```python
from build123d import *


with BuildPart() as f1:
    # F0 (on Front) → F1 (revolve)
    with BuildSketch(Plane.XZ):
        with BuildLine():
            Line((0, 50), (0, 0))
            Line((0, 0), (172.990381, 0))
            Line((172.990381, 0), (160, 7.5))
            Line((160, 7.5), (160, 2.5))
            Line((160, 2.5), (155, 2.5))
            Line((155, 2.5), (22.421579, 75.891626))
            ThreePointArc((22.421579, 75.891626), (17.461092, 75.824589), (15, 71.51716))
            Line((15, 71.51716), (15, 50))
            Line((15, 50), (0, 50))
        make_face()
    revolve(axis=Axis((-26.037737, 0, 0), (-1, 0, 0)))


solid = f1.part
```
Can you work these out from the model? Positions are in its coordinate system, mm. A direction names the side the tool comes from. Coordinates: 2 decimals unless noted, no trailing zeros. Loops run counter-clockwise (first coordinate to the right, second up) from the corner with the lowest first, then second, coordinate; pieces in that order, holes last. Notation, with made-up numbers: (14.5, 69.5) - (20.5, 69.5) arc R11 cw to (20.5, 90.5) - close; hole circle Ø4 at (68, 1.5). An arc over 180 degrees is marked (long way). Answer as CSV lines item,"result". Start each with the question number.
1) Thinking about a two-plate mould opening in X: for faces 1 (the cylindrical face through (7.4, 15.02, 47.69)), 2 (the flat face through (15, 49, 15)), 3 (the flat face through (160, 2, -2)), which applies, pulls with the +X half, pulls with the -X half, needs draft (parallel to the pull), parting line crosses it, or undercut?
2) Which directions (+Z, -Z, +X, -X, +Y, -Y) give clear straight access to the entire face, cutting with the end or side of a thin tool? Please do faces 4 (the flat face through (0, 1, -1)), 5 (the cylindrical face through (157.46, -2.44, -0.54)).
3) Suppose I cut it at B-B (x = 149.5). Please give me the cut outline in (y, z).
4) Suppose I cut it at A-A (x = 56). Please give me the cut outline in (y, z), plus the area to 3 significant figures.
5) For pin 1 (7.5 mm diameter, centred on y = 1, z = -1.5, fed in from -X); pin 2 (1.5 mm diameter, centred on y = -35.5, z = 22, fed in from +X); pin 3 (12 mm diameter, centred on x = 61.5, y = 45, fed in from +Z); pin 4 (1 mm diameter, centred on x = 19.5, z = -45.5, fed in from -Y), each with a flat end and sliding along its axis, tell me the tip position at first contact or that it passes through.
6) I need wall thicknesses on line 1 (Y direction, x = 128, z = -0.5); line 2 (Y direction, x = 38, z = 19); line 3 (Z direction, x = 131, y = -0.5). Which ranges of each line are inside material? Lowest first, please. Write a range as from..to.
Check result:
1,face 1,"needs draft"
1,face 2,"pulls with the -X half"
1,face 3,"undercut"
2,face 4,"+Z, -Z, -X, +Y, -Y"
2,face 5,"none"
3,outline,"circle Ø11.09 at (0, 0)"
4,outline,"circle Ø114.61 at (0, 0)"
4,area,"10,300 mm²"
5,pin 1,"stops at x = 0"
5,pin 2,"stops at x = 85.43"
5,pin 3,"stops at z = 39.35"
5,pin 4,"stops at y = -61.86"
6,line 1,"y = -17.44..17.44"
6,line 2,"y = -64.53..64.53"
6,line 3,"z = -15.78..15.78"
